```python
from build123d import *

# Parameters (mm, degrees)
F1_DEPTH = 5
F2_R     = 3
F3_DEPTH = 5
F4_R     = 3
F5_DEPTH = 5


with BuildPart() as f1:
    # F0 (on Top) → F1 (new body)
    with BuildSketch(Plane.XY):
        with BuildLine():
            ThreePointArc((0, 4), (-4, 0), (0, -4))
            Line((0, -4), (50, -4))
            ThreePointArc((50, -4), (54, 0), (50, 4))
            Line((50, 4), (0, 4))
        make_face()
    extrude(amount=F1_DEPTH)

    # F2 (on face) → F3 (cut, through all)
    with BuildSketch(Plane.XY.offset(5)):
        Circle(F2_R)
    extrude(amount=-F3_DEPTH, mode=Mode.SUBTRACT)

    # F4 (on face) → F5 (cut, through all)
    with BuildSketch(Plane.XY.offset(5)):
        with Locations((50, 0)):
            Circle(F4_R)
    extrude(amount=-F5_DEPTH, mode=Mode.SUBTRACT)


solid = f1.part
```
Work out the finished part from the listing and answer in its coordinate system (mm). Give positions to 0.01 mm unless a question says otherwise; leave off trailing zeros. Write each loop counter-clockwise with the first axis right and the second up, starting at its lowest first coordinate (ties: lowest second). Pieces come first, ordered by that corner, then holes. Notation, with made-up numbers: (79.5, -1) -> (131.5, -1) arc R19 cw to (131.5, 27) -> close; hole circle Ø6 at (83, 74.5). An arc over 180 degrees is marked (long way). Write item = value, one per line.
Q1. Section B-B on z = 3.45 is taken. Determine the outline of the cut face in (x, y).
Computed values:
outline = (0, -4) -> (50, -4) arc R4 ccw to (50, 4) -> (0, 4) arc R4 ccw to start; hole circle Ø6 at (0, 0); hole circle Ø6 at (50, 0)
Q2. Consider line 1 along X through (y, z) = (0.25, 3.95); line 2 along Y through (x, z) = (50, 2.4); line 3 along X through (y, z) = (2.25, 1.7). Determine where each line is inside the solid, lowest interval first.
Computed values:
line_1 = -3.99 to -2.99, 2.99 to 47.01, 52.99 to 53.99
line_2 = -4 to -3, 3 to 4
line_3 = -3.31 to -1.98, 1.98 to 48.02, 51.98 to 53.31
Q3. A flat-ended cylindrical pin translates along its axis: pin 1 Ø1 at (y, z) = (2.5, 2.5) entering from +X. Find the tip coordinate at first contact, or state that the pin passes through.
Computed values:
pin_1 = 53.46
Q4. For a pull along Y with two mould halves and no side action, classify faces 1 (the cylindrical face through (47, 0, 3)), 2 (the flat face through (25, 0, 0)), 3 (the cylindrical face through (-3, 0, 3)), 4 (the cylindrical face through (-4, 0, 2)) as pulls with the +Y half, pulls with the -Y half, needs draft (parallel to the pull), parting line crosses it, or undercut.
Computed values:
face_1 = undercut
face_2 = needs draft
face_3 = undercut
face_4 = parting line crosses it
Q5. Section A-A on y = 0 is taken. Determine the outline of the cut face in (x, z).
Computed values:
outline = (-4, 0) -> (-3, 0) -> (-3, 5) -> (-4, 5) -> close; (3, 0) -> (47, 0) -> (47, 5) -> (3, 5) -> close; (53, 0) -> (54, 0) -> (54, 5) -> (53, 5) -> close
